Design review of the part shown in the three views and the two pictorial views. Dimensions are in mm from the part's minimum x, y and z. A direction names the side the tool comes from. Coordinates: 2 decimals unless noted, no trailing zeros. Write each loop counter-clockwise with the first axis right and the second up, starting at its lowest first coordinate (ties: lowest second). Pieces come first, ordered by that corner, then holes. Notation, with made-up numbers: M -29,-31.75 L 0,-31.75 A18 ccw 0,-27.75 Z; hole C -6,-21 d7. An arc over 180 degrees is marked long. Answer as a JSON object with one key per item and string values.
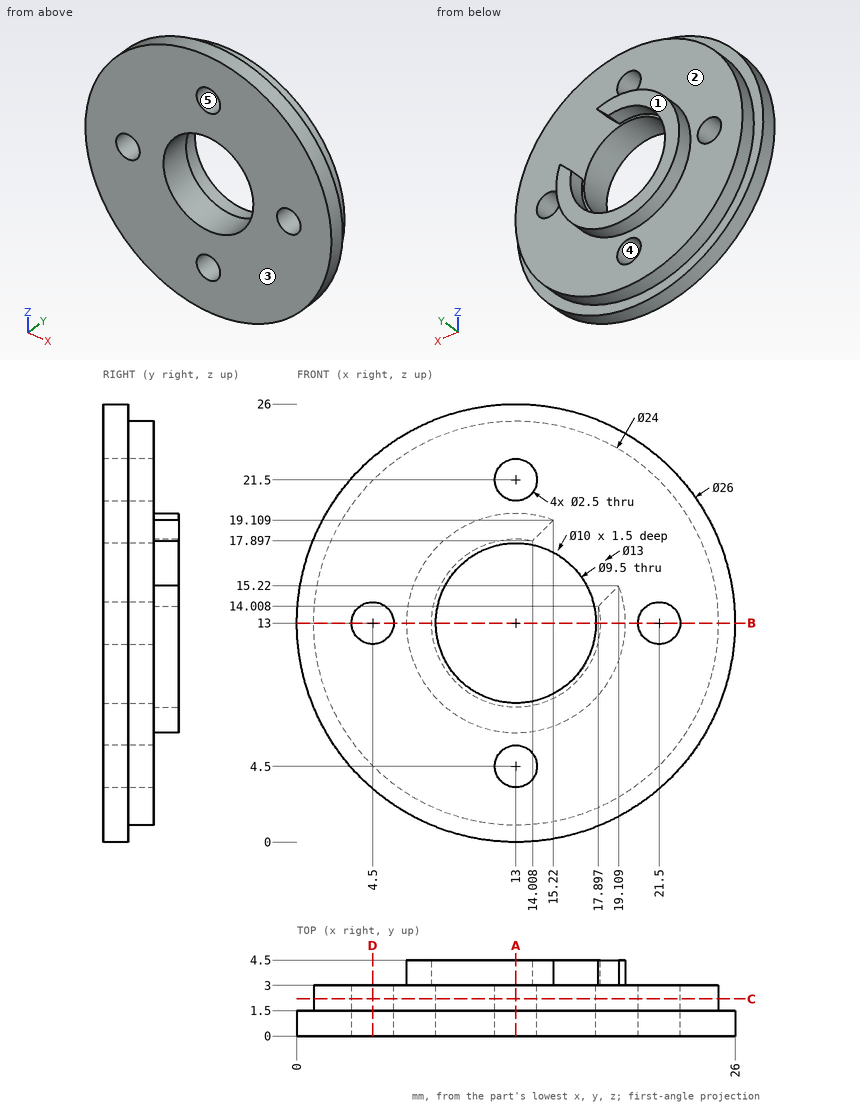
(1) Add section D-D on x = 4.5. Give the boundary of the cut face in (y, z), and give its area (3 significant figures).
Results list:
{"outline": "M 0,3.16 L 1.5,3.16 L 1.5,4.53 L 3,4.53 L 3,11.75 L 0,11.75 Z; M 0,14.25 L 3,14.25 L 3,21.47 L 1.5,21.47 L 1.5,22.84 L 0,22.84 Z", "area": "47.4 mm²"}
(2) For the marked faces 1 and 2, list the 3-axis set-ups (+Z, -Z, +X, -X, +Y, -Y) from which the entire face can be reached by the end or side of a thin tool; tool diameter is ignored.
Results list:
{"face 1": "+Z, -Z, +X, -X, +Y", "face 2": "+Y"}
(3) For pin 1 Ø1.5 at (x, z) = (16, 6) entering from +Y; pin 2 Ø1.5 at (y, z) = (2.5, 10.5) entering from +X; pin 3 Ø1.5 at (y, z) = (3.5, 4.5) entering from +X, all flat-tipped, find the tip position at first contact; note any pin that passes through.
Results list:
{"pin 1": "y = 3", "pin 2": "x = 24.87", "pin 3": "x = 22"}
(4) Add section A-A on x = 13. Give the boundary of the cut face in (y, z), and give its area (3 significant figures).
Results list:
{"outline": "M 0,0 L 1.5,0 L 1.5,1 L 3,1 L 3,3.25 L 0,3.25 Z; M 0,5.75 L 3,5.75 L 3,6.5 L 4.5,6.5 L 4.5,8 L 3,8 L 3,8.25 L 0,8.25 Z; M 0,17.75 L 3,17.75 L 3,18 L 4.5,18 L 4.5,19.5 L 3,19.5 L 3,20.25 L 0,20.25 Z; M 0,22.75 L 3,22.75 L 3,25 L 1.5,25 L 1.5,26 L 0,26 Z", "area": "36.0 mm²"}
(5) Draft analysis for pull direction X (two halves, no side actions). For the marked faces 3, 4 and 5, state which applies: released by +X, released by -X, zero draft, split by the parting line, or undercut.
Results list:
{"face 3": "zero draft", "face 4": "undercut", "face 5": "undercut"}
(6) Wall thickness on line 1 along X through (y, z) = (1.45, 13); line 2 along X through (y, z) = (4.2, 13); line 3 along Z through (x, y) = (13.5, 2.35) (1 decimal): over which ranges is each line inside the solid? List them lowest first. Write a range as from..to.
Results list:
{"line 1": "0..3.25, 5.75..8.25, 17.75..20.25, 22.75..26", "line 2": "6.5..8, 18..19.5", "line 3": "1..3.4, 5.6..8.3, 17.7..20.4, 22.6..25"}
(7) Add section C-C on y = 2.2. Give the boundary of the cut face in (x, z), and give its area (3 significant figures).
Results list:
{"outline": "C 13,13 d24; hole C 4.5,13 d2.5; hole C 13,13 d9.5; hole C 13,4.5 d2.5; hole C 13,21.5 d2.5; hole C 21.5,13 d2.5", "area": "362 mm²"}
(8) Add section B-B on z = 13. Give the boundary of the cut face in (x, y).
Results list:
{"outline": "M 0,0 L 3.25,0 L 3.25,3 L 1,3 L 1,1.5 L 0,1.5 Z; M 5.75,0 L 8.25,0 L 8.25,3 L 8,3 L 8,4.5 L 6.5,4.5 L 6.5,3 L 5.75,3 Z; M 17.75,0 L 20.25,0 L 20.25,3 L 19.5,3 L 19.5,4.5 L 18,4.5 L 18,3 L 17.75,3 Z; M 22.75,0 L 26,0 L 26,1.5 L 25,1.5 L 25,3 L 22.75,3 Z"}
